CAD build for the part. Positions are in the model's coordinates, mm. A direction names the side the tool comes from. Give positions to 0.01 mm unless a question says otherwise; leave off trailing zeros. Order: outer loops, then holes, each group sorted by start corner. A loop starts at its lowest first (then second) coordinate and runs counter-clockwise, first axis right, second up.
from build123d import *

# Parameters (mm, degrees)
F1_DEPTH = 10


# Not quite as in the source:
# - a feature names something its author has since deleted; it is built from what else it names


with BuildPart() as f1:
    # F0 (on Front) → F1 (new body)
    with BuildSketch(Plane.XZ):
        Polygon((235, 50), (250, 50), (250, 70), (260, 70), (260, 90), (250, 90), (250, 110), (0, 110), (0, 90), (-10, 90), (-10, 70), (0, 70), (0, 50), (15, 50), (15, 40), (35, 40), (35, 50), (55, 50), (55, 40), (75, 40), (75, 50), (95, 50), (95, 40), (115, 40), (115, 50), (135, 50), (135, 40), (155, 40), (155, 50), (175, 50), (175, 40), (195, 40), (195, 50), (215, 50), (215, 40), (235, 40), align=None)
    extrude(amount=-F1_DEPTH)


solid = f1.part
1. Wall check: line 1 (X direction, y = 2, z = 45); line 2 (X direction, y = 6.5, z = 92); line 3 (Z direction, x = 130.5, y = 5.5). Give the ranges that are in metal, low to high.
2. Saw through at A-A on x = 201. Give the cut face in (y, z).
3. 3-axis set-ups, long thin cutter, end or side, ignore diameter. For faces 1 (the flat face through (-5, 5, 70)), 2 (the flat face through (55, 5, 45)), 3 (the flat face through (242, 5, 50)), 4 (the flat face through (127, 5, 110)): which of +Z, -Z, +X, -X, +Y, -Y reach the whole face in a straight line?
4. Saw through at B-B on z = 100.5. Give the cut face in (x, y), plus the area to 3 significant figures.
5. Pin check, flat tips, straight feed: P1, Ø5, axis at y = 4, z = 42.5, coming from the -X side; P2, Ø5, axis at x = 121.5, y = 4, coming from the -Z side; P3, Ø3, axis at y = 3, z = 45.5, coming from the +X side. Stop position of each tip, or through.
6. Mould opens along X. For faces 5 (the flat face through (7, 5, 50)), 6 (the flat face through (250, 5, 60)), 7 (the flat face through (35, 5, 45)), 8 (the flat face through (165, 5, 50)) say: released by +X, released by -X, zero draft, split by the parting line, or undercut.
Reported:
1. line 1: x = 15 to 35, 55 to 75, 95 to 115, 135 to 155, 175 to 195, 215 to 235
1. line 2: x = 0 to 250
1. line 3: z = 50 to 110
2. outline: (0, 50) - (10, 50) - (10, 110) - (0, 110) - close
3. face 1: -Z, -X, +Y, -Y
3. face 2: -Z, +Y, -Y
3. face 3: -Z, +X, +Y, -Y
3. face 4: +Z, +X, -X, +Y, -Y
4. outline: (0, 0) - (250, 0) - (250, 10) - (0, 10) - close
4. area: 2,500 mm2
5. P1: stops at x = 15
5. P2: stops at z = 50
5. P3: stops at x = 235
6. face 5: zero draft
6. face 6: released by +X
6. face 7: undercut
6. face 8: undercut
